Design review of the part built by this model. Coordinates are the model's own, in mm. A direction names the side the tool comes from. Round coordinates to 2 decimals unless told otherwise and drop trailing zeros. Write each loop counter-clockwise with the first axis right and the second up, starting at its lowest first coordinate (ties: lowest second). Pieces come first, ordered by that corner, then holes. Notation, with made-up numbers: (55, 69.5) - (69, 69.5) arc R18 ccw to (69, 82.5) - close; hole circle Ø2 at (-28.5, 79.5). An arc over 180 degrees is marked (long way). Use one line per item in the form item = value.
```python
from build123d import *

# Parameters (mm, degrees)
EXTRUDE_THIN1_DEPTH = 1634
CUT_EXTRUDE1_REACH  = 1637.213
SKETCH7_R           = 5


with BuildPart() as part:
    # Sketch6 → Extrude-Thin1 (new body)
    with BuildSketch(Plane(origin=(0, 0, 0), x_dir=(1, 0, 0), z_dir=(0, 1, 0))):
        with BuildLine():
            Line((-23, 35), (-23, -35))
            ThreePointArc((-23, -35), (-20.656854249, -40.656854249), (-15, -43))
            Line((-15, -43), (15, -43))
            ThreePointArc((15, -43), (20.656854249, -40.656854249), (23, -35))
            Line((23, -35), (23, 35))
            ThreePointArc((23, 35), (20.656854249, 40.656854249), (15, 43))
            Line((15, 43), (-15, 43))
            ThreePointArc((-15, 43), (-20.656854249, 40.656854249), (-23, 35))
        make_face()
        with BuildLine():
            Line((-20, 35), (-20, -35))
            ThreePointArc((-20, -35), (-18.535533906, -38.535533906), (-15, -40))
            Line((-15, -40), (15, -40))
            ThreePointArc((15, -40), (18.535533906, -38.535533906), (20, -35))
            Line((20, -35), (20, 35))
            ThreePointArc((20, 35), (18.535533906, 38.535533906), (15, 40))
            Line((15, 40), (-15, 40))
            ThreePointArc((-15, 40), (-18.535533906, 38.535533906), (-20, 35))
        make_face(mode=Mode.SUBTRACT)
    extrude(amount=EXTRUDE_THIN1_DEPTH)

    # Sketch7 → Cut-Extrude1 (cut, up to next)
    with BuildSketch(Plane.ZY.offset(23), mode=Mode.PRIVATE) as cut_extrude1_sk1:
        with Locations((0, 35)):
            Circle(SKETCH7_R)
    cut_extrude1_tool1 = extrude(cut_extrude1_sk1.sketch, amount=-CUT_EXTRUDE1_REACH, mode=Mode.PRIVATE) & part.part
    # Sketch7 → Cut-Extrude1 (cut, up to next)
    with BuildSketch(Plane.ZY.offset(23), mode=Mode.PRIVATE) as cut_extrude1_sk2:
        with Locations((0, 75)):
            Circle(SKETCH7_R)
    cut_extrude1_tool2 = extrude(cut_extrude1_sk2.sketch, amount=-CUT_EXTRUDE1_REACH, mode=Mode.PRIVATE) & part.part
    add(cut_extrude1_tool1.solids().sort_by_distance((-23, 35, 0))[0], mode=Mode.SUBTRACT)
    add(cut_extrude1_tool2.solids().sort_by_distance((-23, 75, 0))[0], mode=Mode.SUBTRACT)


solid = part.part
```
Q1. Machinability: for faces 1 (the flat face through (0, 806, -43)), 2 (the flat face through (-20, 806, 0)), which of the approach directions +Z, -Z, +X, -X, +Y, -Y give a long, thin tool a straight path to every point of the face, cutting with its end or side? Answer none if there is none.
Calculated:
face_1 = -Z, +X, -X, +Y, -Y
face_2 = +Y, -Y
Q2. We need section A-A on x = -6. Write out the cut boundary in (y, z).
Calculated:
outline = (0, -43) - (1634, -43) - (1634, -40) - (0, -40) - close; (0, 40) - (1634, 40) - (1634, 43) - (0, 43) - close
Q3. Draft analysis for pull direction X (two halves, no side actions). For faces 3 (the flat face through (-23, 806, 0)), 4 (the flat face through (0, 806, -40)), 5 (the flat face through (0, 806, 40)), 6 (the flat face through (23, 806, 0)), state which applies: released by +X, released by -X, zero draft, split by the parting line, or undercut.
Calculated:
face_3 = released by -X
face_4 = undercut
face_5 = undercut
face_6 = released by +X
Q4. To check wall thickness, follow line 1 along Y through (x, z) = (-21.15, 0); line 2 along X through (y, z) = (974, -28); line 3 along Z through (x, y) = (15, 1168). State the ranges of each line that lie inside material, in increasing order. Write a range as from..to.
Calculated:
line_1 = 0..30, 40..70, 80..1634
line_2 = -23..-20, 20..23
line_3 = -43..-40, 40..43
Q5. We need section B-B on y = 821.5. Write out the cut boundary in (x, z), then the cut area to 3 significant figures.
Calculated:
outline = (-23, -35) arc R8 ccw to (-15, -43) - (15, -43) arc R8 ccw to (23, -35) - (23, 35) arc R8 ccw to (15, 43) - (-15, 43) arc R8 ccw to (-23, 35) - close; hole (-20, -35) arc R5 ccw to (-15, -40) - (15, -40) arc R5 ccw to (20, -35) - (20, 35) arc R5 ccw to (15, 40) - (-15, 40) arc R5 ccw to (-20, 35) - close
area = 723 mm2
